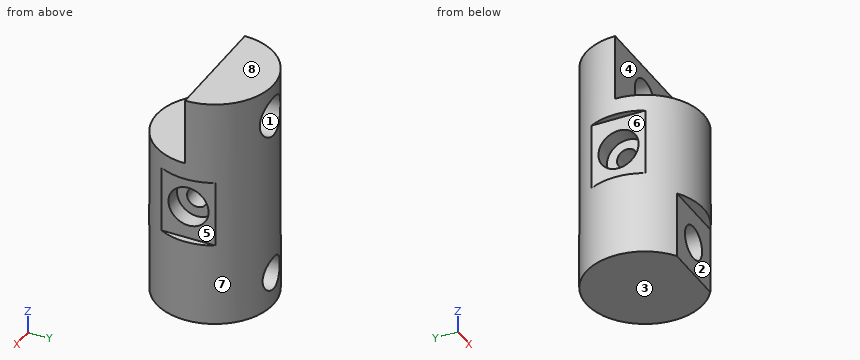
from build123d import *

# Parameters (mm, degrees)
F0_W            = 17.5
F0_H            = 70
F2_W            = 17.5
F2_H            = 20
F3_DEPTH        = 17.501
F3_DEPTH_BACK   = 17.501
F5_D            = 12
F7_START        = 14.5
F6_W            = 35
F6_H            = 20
F7_DEPTH        = 3.0010001
F9_D            = 10
F10_W           = 2
F10_H           = 20
F11_DEPTH       = 17.5010001
F11_DEPTH_BACK  = 17.5010001
F13_D           = 6
F13_CBORE_D     = 12
F13_CBORE_DEPTH = 5


# Not quite as in the source:
# - a pattern or mirror of a feature is missing from the dataset's text; its kind, count and spacing are read off the source's solid


with BuildPart() as f1:
    # F0 (on Front) → F1 (revolve)
    with BuildSketch(Plane.XZ):
        with Locations((8.75, 35)):
            Rectangle(F0_W, F0_H)
    revolve(axis=Axis((0, 0, 35), (0, 0, -1)))

    # F2 (on Right) → F3 (cut, two sides)
    with BuildSketch(Plane.YZ) as f3_sk:
        with Locations((-8.75, 60)):
            Rectangle(F2_W, F2_H)
    extrude(amount=-F3_DEPTH, mode=Mode.SUBTRACT)
    extrude(f3_sk.sketch, amount=F3_DEPTH_BACK, mode=Mode.SUBTRACT)

    # F5 (through all)
    with Locations(Plane.XZ):
        with Locations((0, 60)):
            Hole(F5_D / 2)

    # F6 (on Front) → F7 (cut)
    with BuildSketch(Plane.XZ.offset(F7_START)):
        with Locations((0, 10)):
            Rectangle(F6_W, F6_H)
    extrude(amount=F7_DEPTH, mode=Mode.SUBTRACT)

    # F9 (through all)
    with Locations(Plane.XZ.offset(14.5)):
        with Locations((0, 10)):
            Hole(F9_D / 2)

    # F10 (on Front) → F11 (cut, two sides)
    with BuildSketch(Plane.XZ) as f11_sk:
        with Locations((-16.5, 35)):
            Rectangle(F10_W, F10_H)
        with Locations((16.5, 35)):
            Rectangle(F10_W, F10_H)
    extrude(amount=-F11_DEPTH, mode=Mode.SUBTRACT)
    extrude(f11_sk.sketch, amount=F11_DEPTH_BACK, mode=Mode.SUBTRACT)

    # F13 (through all)
    with Locations(Plane.YZ.offset(15.5)):
        with Locations((0, 35)):
            f13 = CounterBoreHole(F13_D / 2, F13_CBORE_D / 2, F13_CBORE_DEPTH)

    # F13_copies: F13 across plane
    add(f13.mirror(Plane(origin=(0, 0, 0), x_dir=(0, 0, -1), z_dir=(-1, 0, 0))), mode=Mode.SUBTRACT)


solid = f1.part
Geometry check sheet. Reference: the model listing, model coordinates, mm. Face numbers are marked on the shaded views. A direction names the side the tool comes from. Round coordinates to 2 decimals unless told otherwise and drop trailing zeros. Write each loop counter-clockwise with the first axis right and the second up, starting at its lowest first coordinate (ties: lowest second). Pieces come first, ordered by that corner, then holes. Notation, with made-up numbers: (-25.75, 13.25) - (-15.75, 13.25) arc R20 ccw to (-15.75, 32.25) - close; hole circle Ø7 at (61, 41.25). An arc over 180 degrees is marked (long way). One line per item, written item: value.
1. Cross-section at D-D on y = -7. Record the boundary of the cut face in (x, z), and give its area (3 significant figures).
The answers:
outline: (-16.04, 0) - (16.04, 0) - (16.04, 25) - (15.5, 25) - (15.5, 45) - (16.04, 45) - (16.04, 50) - (-16.04, 50) - (-16.04, 45) - (-15.5, 45) - (-15.5, 25) - (-16.04, 25) - close; hole circle Ø10 at (0, 10)
area: 1,500 mm^2
2. Set-up check for the marked faces 4, 5, 6, 7 and 8: record each of +Z, -Z, +X, -X, +Y, -Y from which the full face is reachable in a straight line by a thin tool's end or side.
The answers:
face 4: +Z, +X, -X, -Y
face 5: +X, +Y, -Y
face 6: -X, +Y, -Y
face 7: +Z, -Z
face 8: +Z, +X, -X, +Y, -Y
3. Mould release check, pull along Z, two halves, no side actions. Record for the marked faces 1, 2 and 3: released by +Z, released by -Z, zero draft, split by the parting line, or undercut.
The answers:
face 1: undercut
face 2: zero draft
face 3: released by -Z
4. Cross-section at C-C on y = 1. Record the boundary of the cut face in (x, z).
The answers:
outline: (-17.47, 0) - (17.47, 0) - (17.47, 25) - (15.5, 25) - (15.5, 29.08) - (10.5, 29.08) - (10.5, 32.17) - (-10.5, 32.17) - (-10.5, 29.08) - (-15.5, 29.08) - (-15.5, 25) - (-17.47, 25) - close; (-17.47, 45) - (-15.5, 45) - (-15.5, 40.92) - (-10.5, 40.92) - (-10.5, 37.83) - (10.5, 37.83) - (10.5, 40.92) - (15.5, 40.92) - (15.5, 45) - (17.47, 45) - (17.47, 70) - (-17.47, 70) - close; hole circle Ø12 at (0, 60); hole circle Ø10 at (0, 10)
5. Cross-section at A-A on x = 0. Record the boundary of the cut face in (y, z), and give its area (3 significant figures).
The answers:
outline: (-17.5, 20) - (-14.5, 20) - (-14.5, 15) - (17.5, 15) - (17.5, 54) - (0, 54) - (0, 50) - (-17.5, 50) - close; (-14.5, 0) - (17.5, 0) - (17.5, 5) - (-14.5, 5) - close; (0, 66) - (17.5, 66) - (17.5, 70) - (0, 70) - close; hole circle Ø6 at (0, 35)
area: 1,480 mm^2
6. Depth check by flat-ended pin: pin 1 Ø9.5 at (y, z) = (1.5, 34.5) entering from +X; pin 2 Ø5 at (y, z) = (-3.5, 34.5) entering from -X; pin 3 Ø1.6 at (x, y) = (-17, -2) entering from +Z; pin 4 Ø9.5 at (x, z) = (0, 60) entering from +Y. Enter the tip coordinate at first touch or a pass-through.
The answers:
pin 1: stops at x = 15.5
pin 2: stops at x = -15.5
pin 3: stops at z = 50
pin 4: passes through
7. Scan lines: L1, parallel to Z at x = 0, y = -1; L2, parallel to X at y = 14, z = 27; L3, parallel to Z at x = 0, y = -5.5. Record each from-to range of solid material in increasing order.
The answers:
L1: z = 0 to 5, 15 to 32.17, 37.83 to 50
L2: x = -10.5 to 10.5
L3: z = 0 to 5, 15 to 50
8. Cross-section at B-B on z = 35. Record the boundary of the cut face in (x, y).
The answers:
outline: (-15.5, -8.12) arc R17.5 ccw to (15.5, -8.12) - (15.5, -6) - (10.5, -6) - (10.5, -3) - (-10.5, -3) - (-10.5, -6) - (-15.5, -6) - close; (-15.5, 6) - (-10.5, 6) - (-10.5, 3) - (10.5, 3) - (10.5, 6) - (15.5, 6) - (15.5, 8.12) arc R17.5 ccw to (-15.5, 8.12) - close
